The figure shows three views and two pictorial views of one solid part (mm, origin at its lowest corner). Answer the questions. Give positions to 0.01 mm unless a question says otherwise; leave off trailing zeros. Order: outer loops, then holes, each group sorted by start corner. A loop starts at its lowest first (then second) coordinate and runs counter-clockwise, first axis right, second up. Notation, with made-up numbers: (62, -38.5) -> (72, -38.5) arc R27 cw to (72, -18.5) -> close; hole circle Ø10 at (75, -30.5). An arc over 180 degrees is marked (long way). Use one line per item in the form item = value.
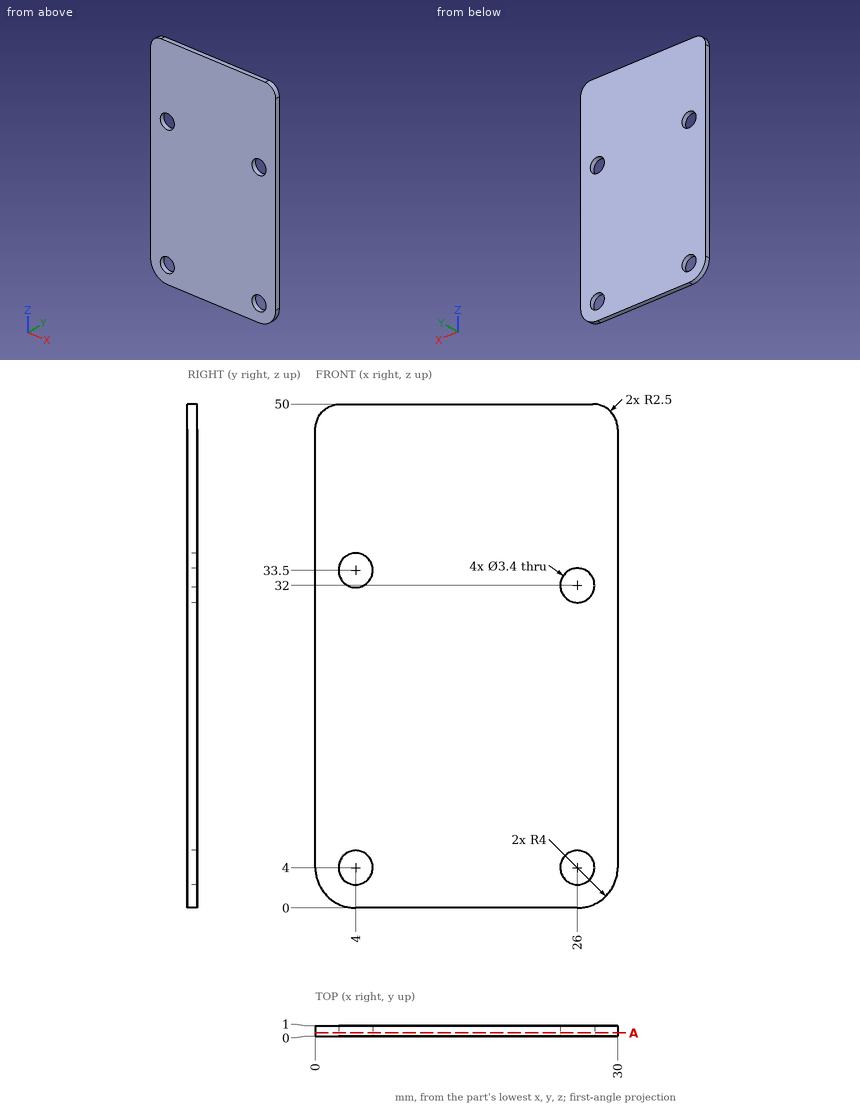
Item 1: Given pin 1 Ø4.5 at (x, z) = (26, 32) entering from -Y; pin 2 Ø3 at (x, z) = (4, 33.5) entering from -Y, each flat-ended and moving along its own axis, determine where each tip first touches the part or whether it passes through.
Checks:
pin_1 = 0
pin_2 = through
Item 2: The part is cut by section A-A on y = 0.3. Give the vertices of the cut face in (x, z).
Checks:
outline = (0, 4) arc R4 ccw to (4, 0) -> (26, 0) arc R4 ccw to (30, 4) -> (30, 47.5) arc R2.5 ccw to (27.5, 50) -> (2.5, 50) arc R2.5 ccw to (0, 47.5) -> close; hole circle Ø3.4 at (4, 4); hole circle Ø3.4 at (4, 33.5); hole circle Ø3.4 at (26, 4); hole circle Ø3.4 at (26, 32)
Item 3: Straight lines are drawn through the part: L1, parallel to Z at x = 4, y = 0.85; L2, parallel to X at y = 0.4, z = 4; L3, parallel to Z at x = 26, y = 0.4. For each, find the intervals that lie inside material, in ascending order. Write a range as from..to.
Checks:
L1 = 0..2.3, 5.7..31.8, 35.2..50
L2 = 0..2.3, 5.7..24.3, 27.7..30
L3 = 0..2.3, 5.7..30.3, 33.7..50
